from build123d import *

# Parameters (mm, degrees)
BASPROSKE_W        = 12.7
BASPROSKE_H        = 7.9375
TOOTHCUT_DEPTH     = 17.949861725
TEETHCUTS_COUNT    = 18
TEETHCUTS_ANGLE    = 340
BORSKE_R           = 3
BORE_DEPTH         = 50.8000508
SKETCH2_R          = 4.5
CUT_EXTRUDE1_DEPTH = 4.95


with BuildPart() as part:
    # BasProSke → Base-Revolve (revolve)
    with BuildSketch(Plane(origin=(0, 0, 0), x_dir=(1, 0, 0), z_dir=(0, 1, 0)), mode=Mode.PRIVATE) as base_revolve_sk:
        with Locations((6.35, 3.96875)):
            Rectangle(BASPROSKE_W, BASPROSKE_H)
    revolve(base_revolve_sk.sketch.rotate(Axis((-10, 0, 0), (1, 0, 0)), 180), axis=Axis((-10, 0, 0), (1, 0, 0)))

    # TooCutSke → ToothCut (cut, through all)
    with BuildSketch(Plane(origin=(0, 0, 0), x_dir=(0, 0, -1), z_dir=(1, 0, 0))):
        with BuildLine():
            ThreePointArc((0.401805019, 6.127289689), (0, 6.14045), (-0.401805019, 6.127289689))
            ThreePointArc((-0.401805019, 6.127289689), (-0.651999955, 7.068698885), (-1.203877601, 7.87136933))
            ThreePointArc((-1.203877601, 7.87136933), (0, 7.9629), (1.203877601, 7.87136933))
            ThreePointArc((1.203877601, 7.87136933), (0.651999955, 7.068698885), (0.401805019, 6.127289689))
        make_face()
    toothcut = extrude(amount=TOOTHCUT_DEPTH, mode=Mode.SUBTRACT)

    # TeethCuts: ToothCut ×18 about axis
    teethcuts_axis = Axis((-10, 0, 0), (1, 0, 0))
    for i in range(1, TEETHCUTS_COUNT):
        add(toothcut.rotate(teethcuts_axis, i * TEETHCUTS_ANGLE / (TEETHCUTS_COUNT - 1)), mode=Mode.SUBTRACT)

    # BorSke → Bore (cut, symmetric)
    with BuildSketch(Plane(origin=(0, 0, 0), x_dir=(0, 0, -1), z_dir=(1, 0, 0))):
        with Locations(Location((0, 0, 0), (0, 0, 180))):
            Circle(BORSKE_R)
    extrude(amount=BORE_DEPTH, both=True, mode=Mode.SUBTRACT)

    # Sketch1 → Revolve1 (revolve)
    with BuildSketch(Plane.XY, mode=Mode.PRIVATE) as revolve1_sk:
        Polygon((12.7, 6.14045), (17.65, 6.46), (17.65, 4.46), (12.7, 4.46), align=None)
    revolve(revolve1_sk.sketch.rotate(Axis((12.7, 0, 0), (1, 0, 0)), 180), axis=Axis((12.7, 0, 0), (1, 0, 0)))

    # Sketch2 → Cut-Extrude1 (cut)
    with BuildSketch(Plane(origin=(17.65, 0, 0), x_dir=(0, 0, -1), z_dir=(1, 0, 0))):
        with Locations(Location((0, 0, 0), (0, 0, 90))):
            Circle(SKETCH2_R)
    extrude(amount=-CUT_EXTRUDE1_DEPTH, mode=Mode.SUBTRACT)


solid = part.part
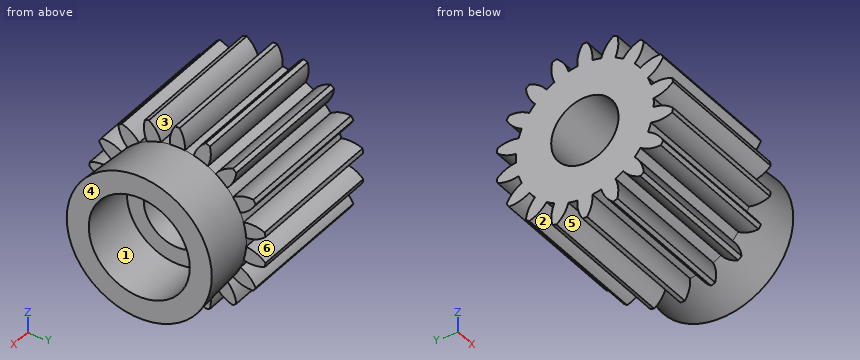
Read the model definition and answer for the solid it produces. Units are mm, in the model's axes. Face numbers are marked on the shaded views. A direction names the side the tool comes from. Round coordinates to 2 decimals unless told otherwise and drop trailing zeros. Order: outer loops, then holes, each group sorted by start corner. A loop starts at its lowest first (then second) coordinate and runs counter-clockwise, first axis right, second up.
1) The mould has two halves that part along Z. Classify the marked faces 4, 5 and 6: released by +Z, released by -Z, zero draft, split by the parting line, or undercut.
2) Straight lines are drawn through the part: L1, parallel to Y at x = 10.75, z = 3.75; L2, parallel to Z at x = 8.5, y = -6; L3, parallel to Z at x = 12, y = 6.75. For each, find the intervals that lie inside material, in ascending order.
3) For the marked faces 1, 2 and 3, determine the directions among +Z, -Z, +X, -X, +Y, -Y from which every point of the face is accessible in a straight line to the end or side of a thin tool.
4) The part is cut by section A-A on z = 0. Write down the section's boundary in (x, y), plus the area to 3 significant figures.
5) Flat-ended cylindrical pins translate along their axes: pin 1 (1 mm diameter, centred on x = 6.5, y = -3, fed in from -Z); pin 2 (1 mm diameter, centred on x = 13.5, y = -5, fed in from -Z); pin 3 (0.7 mm diameter, centred on y = 6.5, z = 1, fed in from +X); pin 4 (2 mm diameter, centred on x = 7.5, y = -4.5, fed in from -Z). Find the tip coordinate at first contact, or state that the pin passes through.
6) The part is cut by section B-B on z = -7. Write down the section's boundary in (x, y), plus the area to 3 significant figures.
Resolved:
1. face 4: zero draft
1. face 5: released by -Z
1. face 6: undercut
2. L1: y = -6.95 to -5.14, -4.86 to 4.86, 5.14 to 6.95
2. L2: z = -4.08 to -2.69, -1.74 to 1.74, 2.69 to 4.08
2. L3: z = -4.14 to -3.42, -1.81 to -0.53, 0.53 to 1.81, 3.42 to 4.14
3. face 1: +X
3. face 2: -Z, -X
3. face 3: +Z, -X
4. outline: (0, -6.14) - (12.7, -6.14) - (17.65, -6.46) - (17.65, -4.5) - (12.7, -4.5) - (12.7, -3) - (0, -3) - close; (0, 3) - (12.7, 3) - (12.7, 4.5) - (17.65, 4.5) - (17.65, 6.46) - (12.7, 6.14) - (0, 6.14) - close
4. area: 97.6 mm2
5. pin 1: stops at z = -7.52
5. pin 2: stops at z = -4.26
5. pin 3: stops at x = 17.65
5. pin 4: stops at z = -6.21
6. outline: (0, -2.97) - (12.7, -2.97) - (12.7, -1.98) - (0, -1.98) - close; (0, -0.6) - (12.7, -0.6) - (12.7, 0.6) - (0, 0.6) - close; (0, 1.98) - (12.7, 1.98) - (12.7, 2.97) - (0, 2.97) - close
6. area: 40.4 mm2
